```python
from build123d import *

# Parameters (mm, degrees)
BOSS_EXTRUDE1_DEPTH = 12.5
BOSS_EXTRUDE2_DEPTH = 4
SKETCH3_R           = 2.3
BOSS_EXTRUDE3_DEPTH = 3.2


with BuildPart() as part:
    # Sketch1 → Boss-Extrude1 (new body)
    with BuildSketch(Plane(origin=(0, 0, 0), x_dir=(1, 0, 0), z_dir=(0, 1, 0))):
        Polygon((0, 17.7), (0, 22.3), (22.6, 22.3), (22.6, 17.7), (27.3, 17.7), (27.3, 15.3), (22.6, 15.3), (22.6, 0), (0, 0), (0, 15.3), (-4.7, 15.3), (-4.7, 17.7), align=None)
    extrude(amount=BOSS_EXTRUDE1_DEPTH)

    # Sketch2 → Boss-Extrude2 (add)
    with BuildSketch(Plane(origin=(0, 0, -22.3), x_dir=(-1, 0, 0), z_dir=(0, 0, -1))):
        with BuildLine():
            ThreePointArc((-10.6, 8.699489743), (-22.6, 6.25), (-10.6, 3.800510257))
            ThreePointArc((-10.6, 3.800510257), (-7.6, 6.25), (-10.6, 8.699489743))
        make_face()
    extrude(amount=BOSS_EXTRUDE2_DEPTH)

    # Sketch3 → Boss-Extrude3 (add)
    with BuildSketch(Plane(origin=(0, 0, -26.3), x_dir=(-1, 0, 0), z_dir=(0, 0, -1))):
        with Locations((-16.35, 6.25)):
            Circle(SKETCH3_R)
    extrude(amount=BOSS_EXTRUDE3_DEPTH)


solid = part.part
```
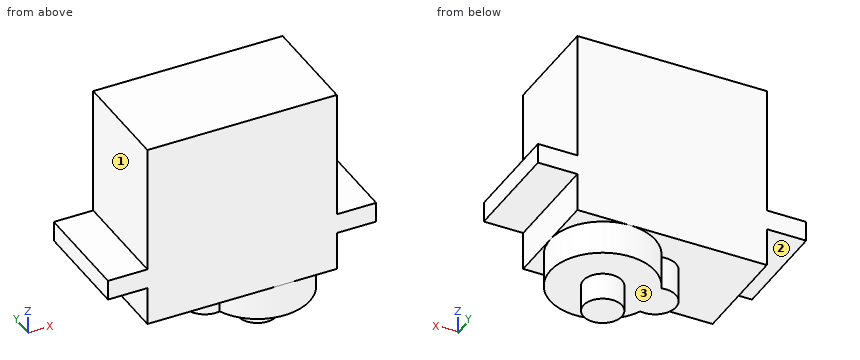
Geometry check sheet. Reference: the model listing, model coordinates, mm. Face numbers are marked on the shaded views. A direction names the side the tool comes from. Coordinates: 2 decimals unless noted, no trailing zeros. Write each loop counter-clockwise with the first axis right and the second up, starting at its lowest first coordinate (ties: lowest second). Pieces come first, ordered by that corner, then holes. Notation, with made-up numbers: M 62.5,-17 L 95.5,-17 A23 ccw 95.5,3 Z; hole C 29.25,30.25 d10. An arc over 180 degrees is marked long. Answer as a JSON object with one key per item and string values.
1. Go/stop test with flat-tipped pins: pin 1 Ø5 at (x, y) = (-3.5, 8) entering from +Z; pin 2 Ø1.9 at (x, y) = (20.5, 3.5) entering from -Z; pin 3 Ø5 at (y, z) = (2.5, -5.5) entering from -X. Record where each tip stops, or that it passes through.
Answers below:
{"pin 1": "stops at z = -15.3", "pin 2": "stops at z = -26.3", "pin 3": "stops at x = 0"}
2. Scan lines: L1, parallel to X at y = 7.25, z = -17.75; L2, parallel to Z at x = 11, y = 4; L3, parallel to Z at x = 24, y = 8. Record each from-to range of solid material in increasing order.
Answers below:
{"L1": "x = 0 to 22.6", "L2": "z = -26.3 to 0", "L3": "z = -17.7 to -15.3"}
3. Section check A-A, the plane x = 10.1. Enter the section's corners in (y, z).
Answers below:
{"outline": "M 0,-22.3 L 3.75,-22.3 L 3.75,-26.3 L 8.75,-26.3 L 8.75,-22.3 L 12.5,-22.3 L 12.5,0 L 0,0 Z"}
4. Section check D-D, the plane x = 17.5. Enter the section's corners in (y, z), plus the area to 3 significant figures.
Answers below:
{"outline": "M 0,-22.3 L 0.11,-22.3 L 0.11,-26.3 L 4.26,-26.3 L 4.26,-29.5 L 8.24,-29.5 L 8.24,-26.3 L 12.39,-26.3 L 12.39,-22.3 L 12.5,-22.3 L 12.5,0 L 0,0 Z", "area": "341 mm²"}
5. Section check B-B, the plane y = 7. Enter the section's corners in (x, z), plus the area to 3 significant figures.
Answers below:
{"outline": "M -4.7,-17.7 L 0,-17.7 L 0,-22.3 L 7.72,-22.3 L 7.72,-26.3 L 14.18,-26.3 L 14.18,-29.5 L 18.52,-29.5 L 18.52,-26.3 L 22.55,-26.3 L 22.55,-22.3 L 22.6,-22.3 L 22.6,-17.7 L 27.3,-17.7 L 27.3,-15.3 L 22.6,-15.3 L 22.6,0 L 0,0 L 0,-15.3 L -4.7,-15.3 Z", "area": "600 mm²"}
6. Tool access check on the marked faces 1, 2 and 3. Record the directions out of +Z, -Z, +X, -X, +Y, -Y that give a thin tool (end or side, any length) a straight path to the whole face; none if there is none.
Answers below:
{"face 1": "+Z, -X, +Y, -Y", "face 2": "-Z, -X, +Y, -Y", "face 3": "-Z"}
7. Section check C-C, the plane z = -13.25. Enter the section's corners in (x, y), plus the area to 4 significant figures.
Answers below:
{"outline": "M 0,0 L 22.6,0 L 22.6,12.5 L 0,12.5 Z", "area": "282.5 mm²"}
